Geometry: final body of the model. Coordinates: model frame, mm. Face numbers are marked on the shaded views. A direction names the side the tool comes from. Give positions to 0.01 mm unless a question says otherwise; leave off trailing zeros. Loops run counter-clockwise (first coordinate to the right, second up) from the corner with the lowest first, then second, coordinate; pieces in that order, holes last. Notation, with made-up numbers: M -16,52.5 L 39,52.5 A11 ccw 39,56.5 Z; hole C 0,-26 d4. An arc over 180 degrees is marked long. Put each result on its own line as item: value.
```python
from build123d import *

# Parameters (mm, degrees)
IZIM1_W                     = 5
IZIM1_H                     = 7
Y_KSEKLIK_EKSTR_ZYON1_DEPTH = 2.8
IZIM2_W                     = 4
IZIM2_H                     = 5
Y_KSEKLIK_EKSTR_ZYON2_DEPTH = 2
RADYUS2_R                   = 2
IZIM3_W                     = 0.7
IZIM3_H                     = 0.7
IZIM5_W                     = 0.7
IZIM5_H                     = 0.7


with BuildPart() as part:
    # Çizim1 → Yükseklik-Ekstrüzyon1 (new body)
    with BuildSketch(Plane.XY):
        with Locations((2.5, 3.5)):
            Rectangle(IZIM1_W, IZIM1_H)
    extrude(amount=Y_KSEKLIK_EKSTR_ZYON1_DEPTH)

    # Çizim2 → Yükseklik-Ekstrüzyon2 (add)
    with BuildSketch(Plane.XY.offset(2.8)):
        with Locations((2.5, 2.5)):
            Rectangle(IZIM2_W, IZIM2_H)
    extrude(amount=Y_KSEKLIK_EKSTR_ZYON2_DEPTH)

    # Radyus2
    radyus2_edges = [part.edges().sort_by_distance(p)[0] for p in [
        (4.5, 2.5, 4.8),
    ]]
    fillet(radyus2_edges, radius=RADYUS2_R - 0.0001)  # a hair under: the kernel refuses the full size
    radyus2_2_edges = [part.edges().sort_by_distance(p)[0] for p in [
        (1.50005, 5, 4.8),
    ]]
    fillet(radyus2_2_edges, radius=RADYUS2_R - 0.0001)  # a hair under: the kernel refuses the full size
    radyus2_3_edges = [part.edges().sort_by_distance(p)[0] for p in [
        (0.5, 1.50005, 4.8),
    ]]
    fillet(radyus2_3_edges, radius=RADYUS2_R - 0.0001)  # a hair under: the kernel refuses the full size

    # Süpür1: sweep along a path in Çizim4
    with BuildLine(Plane(origin=(0, 0, 0.55), x_dir=(-1, 0, 0), z_dir=(0, 0, -1))) as s_p_r1_path:
        Line((-4.2, 0), (-4.2, -1.3))
        Line((-4.2, -1.3), (-5.04, -1.3))
        Line((-5.04, -1.3), (-5.04, -23))
    # Çizim3 → Süpür1 (sweep)
    with BuildSketch(Plane.XZ):
        with Locations((4.2, 0.55)):
            Rectangle(IZIM3_W, IZIM3_H)
    s_p_r1 = sweep(path=s_p_r1_path.line, transition=Transition.RIGHT)

    # Aynalama1: Süpür1 across plane
    add(s_p_r1.mirror(Plane(origin=(2.5, 0, 0), x_dir=(0, 0, 1), z_dir=(1, 0, 0))))

    # Süpür2: sweep along a path in Çizim6
    with BuildLine(Plane(origin=(0, 0, 0.55), x_dir=(-1, 0, 0), z_dir=(0, 0, -1))) as s_p_r2_path:
        Line((-2.5, 0), (-2.5, -23.002662889))
    # Çizim5 → Süpür2 (sweep)
    with BuildSketch(Plane.XZ):
        with Locations((2.5, 0.55)):
            Rectangle(IZIM5_W, IZIM5_H)
    sweep(path=s_p_r2_path.line)


solid = part.part
```
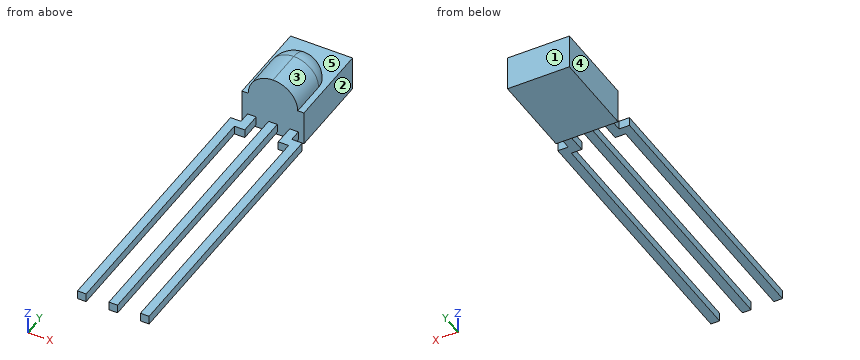
Item 1: Pin query (flat end, axial travel): pin 1 Ø3 at (x, y) = (4.5, -15.5) entering from +Z; pin 2 Ø1.5 at (x, y) = (2, 4.5) entering from +Z; pin 3 Ø0.8 at (x, y) = (0.5, -12) entering from -Z. Return the tip coordinate at first contact, or that it passes through.
Output values:
pin 1: z = 0.9
pin 2: z = 4.62
pin 3: z = 0.2
Item 2: Line query: probe 1 along X at (y, z) = (-15, 0.4); probe 2 along Z at (x, y) = (2.65, -3.5); probe 3 along X at (y, z) = (5.5, 2.15). Output: solid intervals per line, ascending. Write a range as [from, to].
Output values:
probe 1: [-0.39, 0.31], [2.15, 2.85], [4.69, 5.39]
probe 2: [0.2, 0.9]
probe 3: [0, 5]
Item 3: Mould query, pull axis Y, two halves, no side actions, for the marked faces 1 and 2. Classes: pulls with the +Y half, pulls with the -Y half, needs draft (parallel to the pull), parting line crosses it, or undercut.
Output values:
face 1: pulls with the +Y half
face 2: needs draft
Item 4: Set-up query: the marked faces 3, 4 and 5. Return all of +Z, -Z, +X, -X, +Y, -Y with unobstructed straight access to the full face (end or side cutting, diameter ignored); none if empty.
Output values:
face 3: +Z, +X, +Y, -Y
face 4: +Z, -Z, -X, +Y
face 5: +Z, +Y
Item 5: Section C-C on z = 1.7. Output: boundary loops of the cut face in (x, y), then the cut area to 3 significant figures.
Output values:
outline: M 0,0 L 5,0 L 5,7 L 0,7 Z
area: 35.0 mm²
Item 6: Section A-A on y = -21. Output: boundary loops of the cut face in (x, z), then the cut area to 3 significant figures.
Output values:
outline: M -0.39,0.2 L 0.31,0.2 L 0.31,0.9 L -0.39,0.9 Z; M 2.15,0.2 L 2.85,0.2 L 2.85,0.9 L 2.15,0.9 Z; M 4.69,0.2 L 5.39,0.2 L 5.39,0.9 L 4.69,0.9 Z
area: 1.47 mm²
